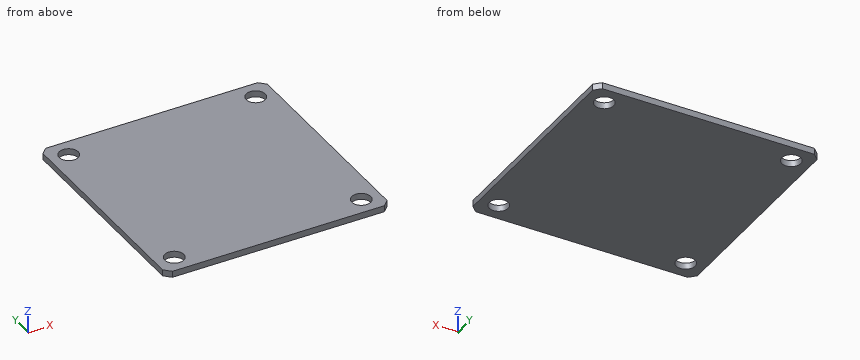
Autodesk Inventor part; units mm, degrees
ref_plane "YZ Plane" through (0, 0, 0) normal (1, 0, 0) x (0, 1, 0)
ref_plane "XZ Plane" through (0, 0, 0) normal (0, 1, 0) x (-1, 0, 0)
ref_plane "XY Plane" through (0, 0, 0) normal (0, 0, 1) x (1, 0, 0)
sketch "Sketch1" plane through (0, 0, 0) normal (0, 0, 1) x (1, 0, 0)
  line L0 (0, 0) -> (36, 0)
  line L1 (36, 0) -> (36, 36)
  line L2 (36, 36) -> (0, 36)
  line L3 (0, 36) -> (0, 0)
  dimension "d0" = 36
  dimension "d1" = 36
extrude "Extrusion1" add sketch "Sketch1" along normal blind 1
sketch "Sketch2" plane through (0, 0, 1) normal (0, 0, 1) x (1, 0, 0)
  line L0 (3, 33) -> (33, 33)
  line L1 (33, 33) -> (33, 3)
  line L2 (33, 3) -> (3, 3)
  line L3 (3, 3) -> (3, 33)
  line L4 (0, 36) -> (0, 0)
  line L5 (36, 36) -> (0, 36)
  circle A0 centre (3, 33) radius 1.525
  circle A1 centre (33, 33) radius 1.525
  circle A2 centre (33, 3) radius 1.525
  circle A3 centre (3, 3) radius 1.525
  dimension "d4" = 30
  dimension "d5" = 30
  dimension "d6" = 3
  dimension "d7" = 3
  dimension "d8" = 3.05
  dimension "d9" = 3.05
  dimension "d10" = 3.05
  dimension "d11" = 3.05
extrude "Extrusion2" cut sketch "Sketch2" against normal through all contours L3 A0 L0 | L0 A0 L3 | A1 L1 L0 | L0 L1 A1 | A3 L2 L3 | L3 L2 A3 | A2 L2 L1 | L1 L2 A2
chamfer "Chamfer1" distance 1 angle 45 4 edges at (0, 36, 0.5) (36, 36, 0.5) (36, 0, 0.5) (0, 0, 0.5)
properties part number "Matek Systems PDU" material "GFRC"
Could you check a few things on this model? Use its own coordinates, in mm. Give positions to 0.01 mm unless a question says otherwise; leave off trailing zeros. Order: outer loops, then holes, each group sorted by start corner. A loop starts at its lowest first (then second) coordinate and runs counter-clockwise, first axis right, second up.
Item 1: I need wall thicknesses on line 1 (X direction, y = 33, z = 0.75) (3 decimals). Which ranges of the line are inside material? Lowest first, please.
Item 2: If we section it at A-A, the plane y = 33: Write out the boundary of the cut face in (x, z) (3 decimals), plus the area to 3 significant figures.
Item 3: I'm going to push a flat-ended pin straight in: pin 1 (3 mm diameter, centred on x = 15.5, y = 24, fed in from -Z). Where does the tip first touch, or does it pass through?
Item 4: If we section it at B-B, the plane z = 0.7: Write out the boundary of the cut face in (x, y) (3 decimals).
Values:
1. line 1: x = 0 to 1.475, 4.525 to 31.475, 34.525 to 36
2. outline: (0, 0) - (1.475, 0) - (1.475, 1) - (0, 1) - close; (4.525, 0) - (31.475, 0) - (31.475, 1) - (4.525, 1) - close; (34.525, 0) - (36, 0) - (36, 1) - (34.525, 1) - close
2. area: 29.9 mm2
3. pin 1: stops at z = 0
4. outline: (0, 1) - (1, 0) - (35, 0) - (36, 1) - (36, 35) - (35, 36) - (1, 36) - (0, 35) - close; hole circle Ø3.05 at (3, 3); hole circle Ø3.05 at (3, 33); hole circle Ø3.05 at (33, 3); hole circle Ø3.05 at (33, 33)
